Check sheet for the modelled part. Datum: model origin and axes. Units: mm. Face numbers are marked on the shaded views. A direction names the side the tool comes from. Give positions to 0.01 mm unless a question says otherwise; leave off trailing zeros. Loops run counter-clockwise (first coordinate to the right, second up) from the corner with the lowest first, then second, coordinate; pieces in that order, holes last. Notation, with made-up numbers: (27, 16.5) -> (69, 16.5) arc R25 ccw to (69, 36.5) -> close; hole circle Ø9 at (88, -19.5). An arc over 180 degrees is marked (long way). Write each question's results on one line, items separated by ' | '. Start each with the question number.
Item 1: Cross-section at B-B on y = 5.5. State how many separate pieces and enclosed holes the cut face has, then the cut area to 3 significant figures.
Item 2: Cross-section at D-D on z = -17. Enter the section's corners in (x, y), then the cut area to 3 significant figures.
Item 3: Scan lines: line 1 along Z through (x, y) = (36, -9); line 2 along Y through (x, z) = (41.5, -18). Record each from-to range of solid material in increasing order.
Item 4: Gauge pin test, flat ends, axial feed: pin 1 Ø6.5 at (x, y) = (38.2, 0) entering from -Z; pin 2 Ø6 at (x, z) = (4.5, -33) entering from -Y. Record the tip position at first contact, or that the pin passes through.
Item 5: Access from +Z, -Z, +X, -X, +Y, -Y to the whole of each face (thin tool, end or side, straight path). Record for the marked faces 1 and 2.
Item 6: Cross-section at A-A on x = 46.5. Enter the section's corners in (y, z), then the cut area to 3 significant figures.
Item 7: Cross-section at C-C on x = -21. Enter the section's corners in (y, z), then the cut area to 3 significant figures.
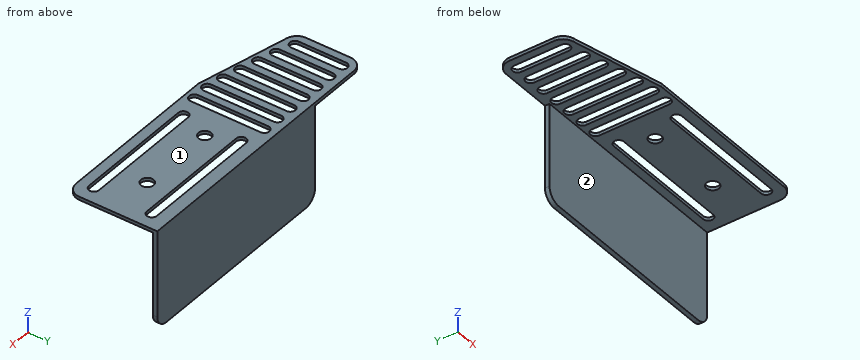
from build123d import *

# Parameters (mm, degrees)
F0_R     = 2.5
F0_W     = 85
F0_H     = 1.8
F1_DEPTH = 1.3
F2_DEPTH = 38
F3_R     = 5


with BuildPart() as f1:
    # F0 (on Top) → F1 (new body)
    with BuildSketch(Plane.XY):
        Polygon((-27.797528, 18), (-53.797528, 18), (-53.797528, -8.664937), (-13.797528, -18), (57.202472, -18), (57.202472, 16.2), (-27.797528, 16.2), align=None)
        with BuildLine():
            Line((-15.797528, -9.769044), (-15.797528, 13.37813))
            ThreePointArc((-15.797528, 13.37813), (-13.797528, 15.37813), (-11.797528, 13.37813))
            Line((-11.797528, 13.37813), (-11.797528, -14.504098))
            ThreePointArc((-11.797528, -14.504098), (-13.797528, -16.504098), (-15.797528, -14.504098))
            Line((-15.797528, -14.504098), (-15.797528, -9.769044))
        make_face(mode=Mode.SUBTRACT)
        with BuildLine():
            Line((-8.797528, -14.504098), (-8.797528, 13.37813))
            ThreePointArc((-8.797528, 13.37813), (-6.797528, 15.37813), (-4.797528, 13.37813))
            Line((-4.797528, 13.37813), (-4.797528, -14.504098))
            ThreePointArc((-4.797528, -14.504098), (-6.797528, -16.504098), (-8.797528, -14.504098))
        make_face(mode=Mode.SUBTRACT)
        with BuildLine():
            ThreePointArc((50.682452, -10), (52.682452, -12), (50.682452, -14))
            Line((50.682452, -14), (2.474277, -14))
            ThreePointArc((2.474277, -14), (0.474277, -12), (2.474277, -10))
            Line((2.474277, -10), (50.682452, -10))
        make_face(mode=Mode.SUBTRACT)
        with BuildLine():
            Line((-50.797528, -5.494929), (-50.797528, 13.37813))
            ThreePointArc((-50.797528, 13.37813), (-48.797528, 15.37813), (-46.797528, 13.37813))
            Line((-46.797528, 13.37813), (-46.797528, -5.494929))
            ThreePointArc((-46.797528, -5.494929), (-48.797528, -7.494929), (-50.797528, -5.494929))
        make_face(mode=Mode.SUBTRACT)
        with BuildLine():
            Line((-43.797528, -7.752692), (-43.797528, 13.37813))
            ThreePointArc((-43.797528, 13.37813), (-41.797528, 15.37813), (-39.797528, 13.37813))
            Line((-39.797528, 13.37813), (-39.797528, -7.752692))
            ThreePointArc((-39.797528, -7.752692), (-41.797528, -9.815282), (-43.797528, -7.752692))
        make_face(mode=Mode.SUBTRACT)
        with BuildLine():
            Line((-36.797528, -9.769044), (-36.797528, 13.37813))
            ThreePointArc((-36.797528, 13.37813), (-34.797528, 15.37813), (-32.797528, 13.37813))
            Line((-32.797528, 13.37813), (-32.797528, -9.769044))
            ThreePointArc((-32.797528, -9.769044), (-34.797528, -11.769044), (-36.797528, -9.769044))
        make_face(mode=Mode.SUBTRACT)
        with BuildLine():
            ThreePointArc((-29.797528, 13.37813), (-27.797528, 15.37813), (-25.797528, 13.37813))
            Line((-25.797528, 13.37813), (-25.768946, -11.704986))
            ThreePointArc((-25.768946, -11.704986), (-27.780942, -13.721572), (-29.797528, -11.709576))
            Line((-29.797528, -11.709576), (-29.797528, 13.37813))
        make_face(mode=Mode.SUBTRACT)
        with BuildLine():
            ThreePointArc((-22.797528, 13.37813), (-20.797528, 15.37813), (-18.797528, 13.37813))
            Line((-18.797528, 13.37813), (-18.797528, -13.363477))
            ThreePointArc((-18.797528, -13.363477), (-20.797528, -15.363477), (-22.797528, -13.363477))
            Line((-22.797528, -13.363477), (-22.797528, 13.37813))
        make_face(mode=Mode.SUBTRACT)
        with Locations((7.202472, 0)):
            Circle(F0_R, mode=Mode.SUBTRACT)
        with Locations((38.202472, 0)):
            Circle(F0_R, mode=Mode.SUBTRACT)
        with BuildLine():
            ThreePointArc((2.474277, 9), (0.474277, 11), (2.474277, 13))
            Line((2.474277, 13), (50.682452, 13))
            ThreePointArc((50.682452, 13), (52.682452, 11), (50.682452, 9))
            Line((50.682452, 9), (2.474277, 9))
        make_face(mode=Mode.SUBTRACT)
        with Locations((14.702472, 17.1)):
            Rectangle(F0_W, F0_H)
    extrude(amount=F1_DEPTH)

    # F0 (on Top) → F2 (join)
    with BuildSketch(Plane.XY):
        with Locations((14.702472, 17.1)):
            Rectangle(F0_W, F0_H)
    extrude(amount=-F2_DEPTH)

    # F3
    f3_edges = [f1.edges().sort_by_distance(p)[0] for p in [
        (-53.797528, 18, 0.65),
        (-53.797528, -8.664937, 0.65),
        (57.202472, -18, 0.65),
        (57.202472, 17.1, -38),
        (-27.797528, 17.1, -38),
    ]]
    fillet(f3_edges, radius=F3_R)


solid = f1.part
Answer sheet:
1) separate pieces: 8 | enclosed holes: 0 | area: 108 mm²
2) outline: (-27.8, 16.2) -> (57.2, 16.2) -> (57.2, 18) -> (-27.8, 18) -> close | area: 153 mm²
3) line 1: z = 0 to 1.3 | line 2: y = 16.2 to 18
4) pin 1: stops at z = 0 | pin 2: stops at y = 16.2
5) face 1: +Z, +X, -X, +Y, -Y | face 2: -Z, +X, -X, -Y
6) outline: (-18, 0) -> (-14, 0) -> (-14, 1.3) -> (-18, 1.3) -> close; (-10, 0) -> (9, 0) -> (9, 1.3) -> (-10, 1.3) -> close; (13, 0) -> (16.2, 0) -> (16.2, -38) -> (18, -38) -> (18, 1.3) -> (13, 1.3) -> close | area: 105 mm²
7) outline: (-16.32, 0) -> (-15.35, 0) -> (-15.35, 1.3) -> (-16.32, 1.3) -> close; (15.37, 0) -> (16.2, 0) -> (16.2, -38) -> (18, -38) -> (18, 1.3) -> (15.37, 1.3) -> close | area: 73.1 mm²
